Here's how the part is built. I have some questions about the finished solid (model axes, mm). Face numbers are marked on the shaded views. A direction names the side the tool comes from. Give positions to 0.01 mm unless a question says otherwise; leave off trailing zeros. Loops run counter-clockwise (first coordinate to the right, second up) from the corner with the lowest first, then second, coordinate; pieces in that order, holes last.
Q1. For the marked faces 5, 6, 7, 8 and 9, which set-ups out of +Z, -Z, +X, -X, +Y, -Y let a thin tool reach every point of the face, with its end or its side?
Q2. Suppose I cut it at A-A (z = 66.5). List the corners of the cut face in (x, y) for me, and give its area (3 significant figures).
Q3. I'm going to push flat-ended pins straight in: P1, Ø10, axis at x = 32.5, z = 86.5, coming from the -Y side; P2, Ø5.5, axis at x = 19, y = 201, coming from the +Z side; P3, Ø17.5, axis at x = 54, y = 16.5, coming from the +Z side; P4, Ø5, axis at y = 68, z = 42.5, coming from the -X side. Where does each tip first touch, or does it pass through?
Q4. Suppose I cut it at C-C (x = -51). List the corners of the cut face in (y, z) for me, and give its area (3 significant figures).
Q5. Thinking about a two-plate mould opening in Y: for the marked faces 1, 2, 3 and 4, which applies, pulls with the +Y half, pulls with the -Y half, needs draft (parallel to the pull), parting line crosses it, or undercut?
Q6. Suppose I cut it at B-B (y = 113.5). List the corners of the cut face in (x, z) for me, and give its area (3 significant figures).
Q7. I need wall thicknesses on probe 1 along Z at (x, y) = (28, 57); probe 2 along Y at (x, z) = (4.5, 49.5); probe 3 along Z at (x, y) = (0, 23). Which ranges of each line are inside material? Lowest first, please.
Q8. Suppose I cut it at D-D (x = 28.5). List the corners of the cut face in (y, z) for me.
```python
from build123d import *

# Parameters (mm, degrees)
F2_DEPTH = 63.5
F3_DEPTH = 273.05
F0_R     = 12.7
F4_DEPTH = 38.1


with BuildPart() as f2:
    # F1 (on Right) → F2 (new body, symmetric)
    with BuildSketch(Plane.YZ):
        Polygon((0, 101.6), (0, 0), (304.8, 0), (304.8, 82.55), (285.75, 97.29961), (273.05, 97.29961), (273.05, 38.1), (38.1, 38.1), (38.1, 101.6), align=None)
    extrude(amount=F2_DEPTH, both=True)

    # F0 (on Front) → F3 (cut)
    with BuildSketch(Plane.XZ):
        Polygon((-12.7, 16.51), (-12.7, 0), (12.7, 0), (12.7, 16.51), (31.75, 16.51), (31.75, 29.21), (12.7, 29.21), (12.7, 38.1), (-12.7, 38.1), (-12.7, 29.21), (-31.75, 29.21), (-31.75, 16.51), align=None)
    extrude(amount=-F3_DEPTH, mode=Mode.SUBTRACT)

    # F0 (on Front) → F4 (cut)
    with BuildSketch(Plane.XZ):
        with BuildLine():
            Line((-63.5, 101.600022), (-63.5, 50.8))
            Line((-63.5, 50.8), (-47.625, 50.8))
            Line((-47.625, 50.8), (-21.093444, 90.350185))
            ThreePointArc((-21.093444, 90.350185), (-11.952951, 98.611784), (0, 101.600022))
            Line((0, 101.600022), (-63.5, 101.600022))
        make_face()
        with BuildLine():
            Line((47.625, 50.8), (63.5, 50.8))
            Line((63.5, 50.8), (63.5, 101.600022))
            Line((63.5, 101.600022), (0, 101.600022))
            ThreePointArc((0, 101.600022), (11.952951, 98.611784), (21.093444, 90.350185))
            Line((21.093444, 90.350185), (47.625, 50.8))
        make_face()
        with Locations((0, 76.2)):
            Circle(F0_R)
    extrude(amount=-F4_DEPTH, mode=Mode.SUBTRACT)


solid = f2.part
```
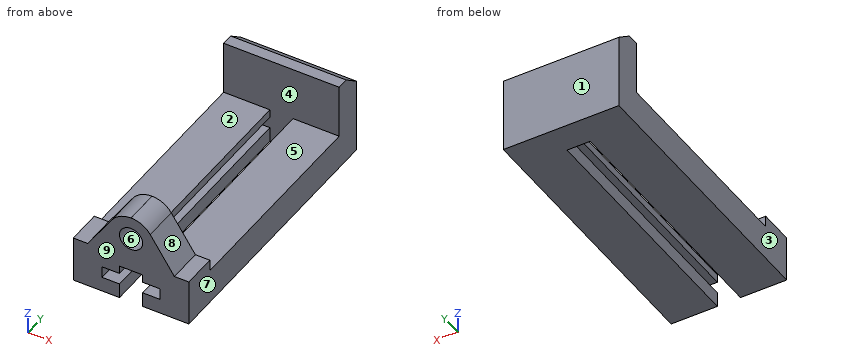
Solutions:
1. face 5: +Z, +X, -X
1. face 6: -Y
1. face 7: +Z, -Z, +X, +Y, -Y
1. face 8: +Z, +X, -Y
1. face 9: +Z, -Z, +X, -X, -Y
2. outline: (-63.5, 273.05) - (63.5, 273.05) - (63.5, 304.8) - (-63.5, 304.8) - close; (-37.09, 0) - (-8.2, 0) - (-8.2, 38.1) - (-37.09, 38.1) - close; (8.2, 0) - (37.09, 0) - (37.09, 38.1) - (8.2, 38.1) - close
2. area: 6,230 mm2
3. P1: stops at y = 273.05
3. P2: stops at z = 38.1
3. P3: stops at z = 54.34
3. P4: passes through
4. outline: (0, 0) - (304.8, 0) - (304.8, 82.55) - (285.75, 97.3) - (273.05, 97.3) - (273.05, 38.1) - (38.1, 38.1) - (38.1, 50.8) - (0, 50.8) - close
4. area: 13,800 mm2
5. face 1: pulls with the +Y half
5. face 2: undercut
5. face 3: needs draft
5. face 4: undercut
6. outline: (-63.5, 0) - (-12.7, 0) - (-12.7, 16.51) - (-31.75, 16.51) - (-31.75, 29.21) - (-12.7, 29.21) - (-12.7, 38.1) - (-63.5, 38.1) - close; (12.7, 0) - (63.5, 0) - (63.5, 38.1) - (12.7, 38.1) - (12.7, 29.21) - (31.75, 29.21) - (31.75, 16.51) - (12.7, 16.51) - close
6. area: 3,390 mm2
7. probe 1: z = 0 to 16.51, 29.21 to 38.1
7. probe 2: y = 0 to 38.1, 273.05 to 304.8
7. probe 3: z = 38.1 to 63.5, 88.9 to 101.6
8. outline: (0, 0) - (304.8, 0) - (304.8, 82.55) - (285.75, 97.3) - (273.05, 97.3) - (273.05, 38.1) - (38.1, 38.1) - (38.1, 79.31) - (0, 79.31) - (0, 29.21) - (273.05, 29.21) - (273.05, 16.51) - (0, 16.51) - close
